from build123d import *

# Parameters (mm, degrees)
F2_SIZE2 = 0.5
F2_SIZE  = 0.5


with BuildPart() as f1:
    # F0 (on Front) → F1 (revolve)
    with BuildSketch(Plane.XZ):
        Polygon((18, 17), (15, 17), (15, 14), (10, 14), (10, 11), (15, 11), (15, 0), (20, 0), (20, 11), (18, 11), align=None)
    revolve(axis=Axis((0, 0, 8.282995), (0, 0, -1)))

    # F2
    f2_edges = [f1.edges().sort_by_distance(p)[0] for p in [
        (-15, 0, 17),
        (-10, 0, 14),
        (-15, 0, 11),
        (-15, 0, 0),
        (-20, 0, 11),
        (-18, 0, 17),
        (-20, 0, 0),
    ]]
    chamfer(f2_edges, length=F2_SIZE, length2=F2_SIZE2)


solid = f1.part
Could you check a few things on this model? Use its own coordinates, in mm. A direction names the side the tool comes from. Give positions to 0.01 mm unless a question says otherwise; leave off trailing zeros. Return JSON: item names as keys, results as strings.
1. I need wall thicknesses on line 1 (Y direction, x = -0.5, z = 8.75); line 2 (Y direction, x = 0, z = 14.7). Which ranges of each line are inside material? Lowest first, please. Write a range as from..to.
Answer list:
{"line 1": "y = -19.99..-14.99, 14.99..19.99", "line 2": "y = -18..-15, 15..18"}
2. On a 3-axis mill with a long thin cutter (end or side, diameter ignored), from which of +Z, -Z, +X, -X, +Y, -Y can I reach the whole of each face in a straight line? I mean faces 1 (the cylindrical face through (-14.985, -0.66, 15.232)), 2 (the flat face through (-3, -10, 11)), 3 (the cylindrical face through (-4.336, 19.524, 5.57)). Say none if no direction works.
Answer list:
{"face 1": "+Z", "face 2": "-Z", "face 3": "+Z, -Z"}
3. Thinking about a two-plate mould opening in X: for faces 4 (the flat face through (-7, 14, 17)), 5 (the cylindrical face through (-2.343, -17.847, 13.788)), 6 (the flat face through (3.1, -10.2, 14)), which applies, pulls with the +X half, pulls with the -X half, needs draft (parallel to the pull), parting line crosses it, or undercut?
Answer list:
{"face 4": "needs draft", "face 5": "parting line crosses it", "face 6": "undercut"}
4. For pin 1 Ø8.5 at (x, y) = (-1.5, 3) entering from -Z; pin 2 Ø8 at (y, z) = (12, 2) entering from -X; pin 3 Ø4 at (y, z) = (-6, 5.5) entering from -X; pin 4 Ø2 at (y, z) = (-11, 9.5) entering from -X, each with a flat end and sliding along its axis, tell me the tip position at first contact or that it passes through.
Answer list:
{"pin 1": "passes through", "pin 2": "stops at x = -18.33", "pin 3": "stops at x = -19.6", "pin 4": "stops at x = -17.32"}
